The listing builds one solid part. Answer for the finished solid, in the listing's coordinates (mm). A direction names the side the tool comes from. Coordinates: 2 decimals unless noted, no trailing zeros. Order: outer loops, then holes, each group sorted by start corner. A loop starts at its lowest first (then second) coordinate and runs counter-clockwise, first axis right, second up.
from build123d import *

# Parameters (mm, degrees)
SKETCH1_R           = 22.5
BOSS_EXTRUDE1_DEPTH = 162
SKETCH4_R           = 22.5
SKETCH4_R_2         = 15
CUT_EXTRUDE1_DEPTH  = 91
SKETCH5_R           = 15
CUT_EXTRUDE2_DEPTH  = 45
SKETCH12_R          = 10
CUT_EXTRUDE3_DEPTH  = 118
SKETCH13_W          = 3
SKETCH13_H          = 3
CUT_EXTRUDE4_DEPTH  = 50


with BuildPart() as part:
    # Sketch1 → Boss-Extrude1 (new body)
    with BuildSketch(Plane.XY):
        Circle(SKETCH1_R)
    extrude(amount=BOSS_EXTRUDE1_DEPTH)

    # Sketch3 → Revolve1 (revolve)
    with BuildSketch(Plane(origin=(0, 0, 0), x_dir=(0, 0, -1), z_dir=(1, 0, 0))):
        Polygon((-157, 110), (-162, 110), (-162, 109.592881079), (-152, 48.592881079), (-152, 22.5), (-147, 22.5), (-147, 49), align=None)
    revolve(axis=Axis((0, 0, 162), (0, 0, -1)))

    # Sketch4 → Cut-Extrude1 (cut)
    with BuildSketch(Plane(origin=(0, 0, 0), x_dir=(-1, 0, 0), z_dir=(0, 0, -1))):
        Circle(SKETCH4_R)
        Circle(SKETCH4_R_2, mode=Mode.SUBTRACT)
    extrude(amount=-CUT_EXTRUDE1_DEPTH, mode=Mode.SUBTRACT)

    # Sketch5 → Cut-Extrude2 (cut)
    with BuildSketch(Plane(origin=(0, 0, 0), x_dir=(-1, 0, 0), z_dir=(0, 0, -1))):
        Circle(SKETCH5_R)
    extrude(amount=-CUT_EXTRUDE2_DEPTH, mode=Mode.SUBTRACT)

    # Sketch12 → Cut-Extrude3 (cut, through all)
    with BuildSketch(Plane(origin=(0, 0, 45), x_dir=(-1, 0, 0), z_dir=(0, 0, -1))):
        Circle(SKETCH12_R)
    extrude(amount=-CUT_EXTRUDE3_DEPTH, mode=Mode.SUBTRACT)

    # Sketch13 → Cut-Extrude4 (cut)
    with BuildSketch(Plane(origin=(0, 0, 45), x_dir=(-1, 0, 0), z_dir=(0, 0, -1))):
        with Locations((0, -10)):
            Rectangle(SKETCH13_W, SKETCH13_H)
    extrude(amount=-CUT_EXTRUDE4_DEPTH, mode=Mode.SUBTRACT)


solid = part.part
1) A tool of negligible diameter and unlimited length cuts with its end or side. For faces 1 (the face through (-5, -15, 91)), 2 (the face through (-10, 21, 152)), 3 (the face through (5, -10, 162)), from which of +Z, -Z, +X, -X, +Y, -Y can it reach the whole face along a straight path? Write none if from no direction.
2) Section C-C (z = 130) is taken. Give the vertices of the cut face in (x, y), then the cut area to 3 significant figures.
3) Consider L1, parallel to Y at x = 0, z = 128; L2, parallel to Y at x = 0, z = 85; L3, parallel to Z at x = 34, y = 12. Determine where each line is inside the solid, lowest interval first.
4) Determine the mould class of faces 4 (the face through (-107.384, -23.846, 159.535)), 5 (the face through (-10, -21, 147)), 6 (the face through (-19.746, 47.624, 152.486)) for opening direction X: released by +X, released by -X, zero draft, split by the parting line, or undercut.
5) Section B-B (z = 57) is taken. Give the vertices of the cut face in (x, y).
6) Each of these flat-tipped pins is pushed along its axis until it touches: P1, Ø6, axis at x = 10.5, z = 57.5, coming from the -Y side; P2, Ø12, axis at x = -75.5, y = -63.5, coming from the -Z side; P3, Ø10, axis at x = -13.5, y = -69, coming from the +Z side. Where does it stop, or does it pass through?
7) Section A-A (y = 0) is taken. Give the vertices of the cut face in (x, z), then the cut area to 3 significant figures.
Filled sheet:
1. face 1: -Z
1. face 2: +Z
1. face 3: +Z, +X, -X, +Y, -Y
2. outline: circle Ø45 at (0, 0); hole circle Ø20 at (0, 0)
2. area: 1,280 mm2
3. L1: y = -22.5 to -10, 10 to 22.5
3. L2: y = -15 to -11.5, 10 to 15
3. L3: z = 147 to 152
4. face 4: split by the parting line
4. face 5: zero draft
4. face 6: undercut
5. outline: circle Ø30 at (0, 0); hole (-1.5, -11.5) - (1.5, -11.5) - (1.5, -9.89) arc R10 ccw (long way) to (-1.5, -9.89) - close
6. P1: stops at y = -12.99
6. P2: stops at z = 154.16
6. P3: stops at z = 156.38
7. outline: (-110, 157) - (-49, 147) - (-22.5, 147) - (-22.5, 91) - (-15, 91) - (-15, 45) - (-10, 45) - (-10, 162) - (-22.5, 162) - (-22.5, 152) - (-48.59, 152) - (-109.59, 162) - (-110, 162) - close; (10, 45) - (15, 45) - (15, 91) - (22.5, 91) - (22.5, 147) - (49, 147) - (110, 157) - (110, 162) - (109.59, 162) - (48.59, 152) - (22.5, 152) - (22.5, 162) - (10, 162) - close
7. area: 3,120 mm2
